Part model, mm, in its own coordinate system. A direction names the side the tool comes from. Coordinates: 2 decimals unless noted, no trailing zeros. Order: outer loops, then holes, each group sorted by start corner. A loop starts at its lowest first (then second) coordinate and runs counter-clockwise, first axis right, second up. Notation, with made-up numbers: (16, 49.5) - (21, 49.5) arc R15 ccw to (21, 66.5) - close; hole circle Ø9 at (75.25, -27). An arc over 180 degrees is marked (long way). Use a Markdown table: item, result. Add a question column.
1) Saw through at B-B on x = -7.5. Count the separate pieces of the cut face and the enclosed holes in it, then the cut area to 3 significant figures.
2) Tool access for faces 4 (the face through (53.57, -12.04, 41.07)), 5 (the face through (67.487, -29.584, -1.344)), 6 (the face through (10, -26, -72)): list every direction of +Z, -Z, +X, -X, +Y, -Y with a clear straight run to the whole face (end or side of a thin tool).
3) Wall check: L1, parallel to Z at x = 0, y = -21; L2, parallel to Z at x = 40, y = -24.5; L3, parallel to X at y = -25.5, z = 45. Give the ranges that are in metal, low to high. Write a range as [from, to].
4) Drop flat-ended pins along their axis: P1, Ø3.5, axis at y = -28, z = -74, coming from the -X side; P2, Ø12, axis at y = -10.5, z = 51, coming from the +X side; P3, Ø5, axis at y = -29.51, z = 72.31, coming from the +X side; P4, Ø5, axis at y = -31.5, z = -9.5, coming from the -X side. Give the stop position or say it passes through.
5) Saw through at A-A on z = 0. List the corners of the cut face in (x, y).
6) Two-plate mould, pull along Y, no slides. Class faces 1 (the face through (0.14, -28.606, 69.446)), 2 (the face through (4.94, -27.401, 78.344)), 3 (the face through (-20, 0, 60)): +Y half, -Y half, draft (parallel to the pull), parting line (faces both ways), or undercut.
Autodesk Inventor part; units mm, degrees
ref_plane "Work Plane1" through (0, -4.0037, -78.5) normal (0, 0, -1) x (-1, 0, 0)
ref_plane "Work Plane2" through (0, -20.011, 78.5) normal (0, 0, 1) x (1, 0, 0)
ref_plane "YZ Plane" through (0, 0, 0) normal (1, 0, 0) x (0, 1, 0)
sketch "Sketch1" plane through (0, 0, 0) normal (0, 0, 1) x (1, 0, 0)
  line L0 (0, 0) -> (-171.0711, 0) construction
  line L1 (0, 0) -> (0, -629.6601) construction
  line L2 (-62.5, 0) -> (-62.5, -35)
  line L3 (-62.5, -35) -> (-67.5, -35)
  line L4 (-62.5, 0) -> (-67.5, 0)
  line L5 (-67.5, 0) -> (-78.5, -4.0037)
  line L6 (-78.5, -4.0037) -> (-78.5, -6.0037)
  line L7 (-78.5, -6.0037) -> (-67.5, -10.0073)
  line L8 (-67.5, -10.0073) -> (-67.5, -14.0073)
  line L9 (-67.5, -14.0073) -> (-78.5, -18.011)
  line L10 (-78.5, -18.011) -> (-78.5, -20.011)
  line L11 (-67.5, -35) -> (-67.5, 0) construction
  line L12 (-78.5, -20.011) -> (-67.5, -24.0147)
  line L13 (-78.5, -20.011) -> (-66.794, -20.011) construction
  line L14 (-67.5, -24.0147) -> (-67.5, -35)
  line L15 (-62.5, -33.4145) -> (-62.8994, -35)
  dimension "d1" = 35
  dimension "d2" = 5
  dimension "d3" = 5
  dimension "d6" = 2
  dimension "d8" = 2
  dimension "d10" = 40
  dimension "d11" = 62.5
  dimension "d12" = 20
  dimension "d13" = 4
  dimension "d14" = 11
  dimension "d15" = 5
revolve "Revolution1" add sketch "Sketch1" angle 360 about axis through (0, 0, 0) along (0, -1, 0)
sketch "Sketch2" plane through (0, 0, 0) normal (0, 0, 1) x (1, 0, 0)
  point P0 (0, 0)
sketch "Sketch3" plane through (0, 0, 0) normal (1, 0, 0) x (0, 1, 0)
  line L0 (-6.0037, -78.5) -> (-4.0037, -78.5)
  line L1 (-20.011, -78.5) -> (-18.011, -78.5)
  line L2 (-4.0037, -78.5) -> (-20.011, -78.5)
  line L3 (-6.0037, -78.5) -> (-6.0037, 78.5)
  line L4 (-6.0037, 78.5) -> (-4.0037, 78.5)
  line L5 (-20.011, 78.5) -> (-18.011, 78.5)
  line L6 (-20.011, -78.5) -> (-20.011, 78.5)
  line L7 (-20.011, 78.5) -> (-4.0037, 78.5)
  point P0 (0, 0)
ref_plane "Work Plane1" through (0, -4.0037, -78.5) normal (0, 0, -1) x (-1, 0, 0)
sketch "Sketch4" plane through (0, -4.0037, -78.5) normal (0, 0, -1) x (-1, 0, 0)
  line L0 (67.5, -30.9963) -> (-67.5, -30.9963)
  line L1 (10, -30.9963) -> (-10, -30.9963)
  line L2 (-10, -30.9963) -> (-10, -16.0073)
  line L3 (-10, -16.0073) -> (10, -16.0073)
  line L4 (10, -16.0073) -> (10, -30.9963)
  line L5 (0, 0) -> (0, -16.0073)
  point P0 (0, 4.0037)
  dimension "d17" = 20
  dimension "d18" = 10
ref_plane "Work Plane2" through (0, -20.011, 78.5) normal (0, 0, 1) x (1, 0, 0)
extrude "Extrusion1" add sketch "Sketch4" against normal up to surface (157 mm away)
sketch "Sketch5" plane through (0, -20.011, 0) normal (0, 1, 0) x (1, 0, 0)
  circle A0 centre (0, 0) radius 62.5
  arc A1 (-10, -61.6948) -> (10, -61.6948) centre (0, 0) ccw
  line L0 (10, 61.6948) -> (10, -61.6948)
  arc A2 (10, 61.6948) -> (-10, 61.6948) centre (0, 0) ccw
  line L1 (-10, 61.6948) -> (-10, -61.6948)
  arc A3 (-10, -77.8605) -> (0, -78.5) centre (0, 0) ccw
  line L2 (-10, -77.8605) -> (-10, -78.5)
  line L3 (-10, -78.5) -> (0, -78.5)
  arc A4 (0, -78.5) -> (10, -77.8605) centre (0, 0) ccw
  line L4 (0, -78.5) -> (10, -78.5)
  line L5 (10, -77.8605) -> (10, -78.5)
  arc A5 (0, 78.5) -> (-10, 77.8605) centre (0, 0) ccw
  line L6 (-10, 78.5) -> (0, 78.5)
  line L7 (-10, 78.5) -> (-10, 77.8605)
  arc A6 (10, 77.8605) -> (0, 78.5) centre (0, 0) ccw
  line L8 (10, 78.5) -> (10, 77.8605)
  line L9 (0, 78.5) -> (10, 78.5)
  point P0 (0, -78.5)
  point P1 (0, -78.5)
  point P2 (0, -78.5)
  point P3 (0, -78.5)
  point P4 (-10, 61.6948)
  point P5 (-10, -61.6948)
  point P6 (10, -61.6948)
extrude "Extrusion2" cut sketch "Sketch5" against normal through all contours L0 A0 L1 | A4 L5 L4 | A3 L3 L2 | A5 L7 L6 | L9 L8 A6
sketch "Sketch6" plane through (10, -35, -77.8605) normal (1, 0, 0) x (0, 0, -1)
  line L0 (0, 0) -> (0.6395, 0) construction
  line L1 (-11.1053, 10.9853) -> (-11.1053, 0) construction
  line L2 (0.6395, 0) -> (-11.1053, 10.9853) construction
  circle A0 centre (-5.2329, 5.4927) radius 3
  line L3 (-144.6156, 10.9853) -> (-144.6156, 0) construction
  line L4 (-155.7209, 14.989) -> (-155.7209, 0) construction
  line L5 (-144.6156, 10.9853) -> (-155.7209, 0) construction
  circle A1 centre (-150.1683, 5.4927) radius 3
  point P0 (-77.8605, 35)
  dimension "d23" = 6
  dimension "d24" = 6
extrude "Extrusion3" cut sketch "Sketch6" against normal through all
properties part number "adapter_za_motor"
Results are:
| question | item | result |
|---|---|---|
| 1 | separate pieces | 2 |
| 1 | enclosed holes | 2 |
| 1 | area | 849 mm2 |
| 2 | face 4 | none |
| 2 | face 5 | +X, -Y |
| 2 | face 6 | -Z, +X, -Y |
| 3 | L1 | [-78.5, -62.5], [62.5, 78.5] |
| 3 | L2 | [-54.37, -48.02], [48.02, 54.37] |
| 3 | L3 | [-50.31, -43.37], [43.37, 50.31] |
| 4 | P1 | x = -10 |
| 4 | P2 | x = 62.85 |
| 4 | P3 | through |
| 4 | P4 | x = -67.14 |
| 5 | outline | (-78.5, -20.01) - (-67.5, -24.01) - (-67.5, -35) - (-62.5, -35) - (-62.5, 0) - (-67.5, 0) - (-78.5, -4) - (-78.5, -6) - (-67.5, -10.01) - (-67.5, -14.01) - (-78.5, -18.01) - close; (62.5, -35) - (67.5, -35) - (67.5, -24.01) - (78.5, -20.01) - (78.5, -18.01) - (67.5, -14.01) - (67.5, -10.01) - (78.5, -6) - (78.5, -4) - (67.5, 0) - (62.5, 0) - close |
| 6 | face 1 | undercut |
| 6 | face 2 | draft |
| 6 | face 3 | +Y half |
